```python
from build123d import *

# Parameters (mm, degrees)
F0_W     = 111
F0_H     = 68.5
F0_W_2   = 108
F0_H_2   = 65.5
F0_R     = 2.5
F0_R_2   = 1.25
F1_DEPTH = 1.5
F2_DEPTH = 13
F3_DEPTH = 8


with BuildPart() as f1:
    # F0 (on Top) → F1 (new body)
    with BuildSketch(Plane.XY):
        with Locations((-16, 1.25)):
            Rectangle(F0_W, F0_H)
        with Locations((-16, 1.25)):
            Rectangle(F0_W_2, F0_H_2, mode=Mode.SUBTRACT)
        with Locations((-16, 1.25)):
            Rectangle(F0_W_2, F0_H_2)
        with Locations((-34, -10.5)):
            Circle(F0_R, mode=Mode.SUBTRACT)
        with Locations((34, -10.5)):
            Circle(F0_R, mode=Mode.SUBTRACT)
        with Locations((-34, 27.1)):
            Circle(F0_R, mode=Mode.SUBTRACT)
        with Locations((34, 27.1)):
            Circle(F0_R, mode=Mode.SUBTRACT)
        with Locations((-34, -10.5)):
            Circle(F0_R)
        with Locations((-34, -10.5)):
            Circle(F0_R_2, mode=Mode.SUBTRACT)
        with Locations((-34, -10.5)):
            Circle(F0_R_2)
        with Locations((34, -10.5)):
            Circle(F0_R)
        with Locations((34, -10.5)):
            Circle(F0_R_2, mode=Mode.SUBTRACT)
        with Locations((34, -10.5)):
            Circle(F0_R_2)
        with Locations((34, 27.1)):
            Circle(F0_R)
        with Locations((34, 27.1)):
            Circle(F0_R_2, mode=Mode.SUBTRACT)
        with Locations((34, 27.1)):
            Circle(F0_R_2)
        with Locations((-34, 27.1)):
            Circle(F0_R)
        with Locations((-34, 27.1)):
            Circle(F0_R_2, mode=Mode.SUBTRACT)
        with Locations((-34, 27.1)):
            Circle(F0_R_2)
    extrude(amount=-F1_DEPTH)

    # F0 (on Top) → F2 (join)
    with BuildSketch(Plane.XY):
        with Locations((-16, 1.25)):
            Rectangle(F0_W, F0_H)
        with Locations((-16, 1.25)):
            Rectangle(F0_W_2, F0_H_2, mode=Mode.SUBTRACT)
        with Locations((-34, 27.1)):
            Circle(F0_R_2)
        with Locations((34, 27.1)):
            Circle(F0_R_2)
        with Locations((34, -10.5)):
            Circle(F0_R_2)
        with Locations((-34, -10.5)):
            Circle(F0_R_2)
    extrude(amount=F2_DEPTH)

    # F0 (on Top) → F3 (join)
    with BuildSketch(Plane.XY):
        with Locations((-34, 27.1)):
            Circle(F0_R)
        with Locations((-34, 27.1)):
            Circle(F0_R_2, mode=Mode.SUBTRACT)
        with Locations((-34, -10.5)):
            Circle(F0_R)
        with Locations((-34, -10.5)):
            Circle(F0_R_2, mode=Mode.SUBTRACT)
        with Locations((34, 27.1)):
            Circle(F0_R)
        with Locations((34, 27.1)):
            Circle(F0_R_2, mode=Mode.SUBTRACT)
        with Locations((34, -10.5)):
            Circle(F0_R)
        with Locations((34, -10.5)):
            Circle(F0_R_2, mode=Mode.SUBTRACT)
    extrude(amount=F3_DEPTH)


solid = f1.part
```
Geometry: final body of the model. Coordinates: model frame, mm. A direction names the side the tool comes from. Coordinates: 2 decimals unless noted, no trailing zeros. Order: outer loops, then holes, each group sorted by start corner. A loop starts at its lowest first (then second) coordinate and runs counter-clockwise, first axis right, second up. Notation, with made-up numbers: (-15.75, -2) - (18.25, -2) arc R8 cw to (18.25, 9) - close; hole circle Ø3 at (73, 61). An arc over 180 degrees is marked (long way). Write each question's results on one line, items separated by ' | '.
(1) Section query D-D, the plane y = -10.5. Return the cut outline in (x, z), plus the area to 4 significant figures.
Values found:
outline: (-71.5, -1.5) - (39.5, -1.5) - (39.5, 13) - (38, 13) - (38, 0) - (36.5, 0) - (36.5, 8) - (35.25, 8) - (35.25, 13) - (32.75, 13) - (32.75, 8) - (31.5, 8) - (31.5, 0) - (-31.5, 0) - (-31.5, 8) - (-32.75, 8) - (-32.75, 13) - (-35.25, 13) - (-35.25, 8) - (-36.5, 8) - (-36.5, 0) - (-70, 0) - (-70, 13) - (-71.5, 13) - close | area: 310.5 mm²
(2) Section query C-C, the plane x = -34. Return the cut outline in (y, z), plus the area to 3 significant figures.
Values found:
outline: (-33, -1.5) - (35.5, -1.5) - (35.5, 13) - (34, 13) - (34, 0) - (29.6, 0) - (29.6, 8) - (28.35, 8) - (28.35, 13) - (25.85, 13) - (25.85, 8) - (24.6, 8) - (24.6, 0) - (-8, 0) - (-8, 8) - (-9.25, 8) - (-9.25, 13) - (-11.75, 13) - (-11.75, 8) - (-13, 8) - (-13, 0) - (-31.5, 0) - (-31.5, 13) - (-33, 13) - close | area: 247 mm²
(3) First-contact query: pin 1 Ø1.5 at (x, y) = (16, 19.5) entering from +Z; pin 2 Ø1.5 at (x, y) = (-34.5, 28.5) entering from +Z. Flat tips, straight axial feed; report the tip coordinate or a pass-through.
Values found:
pin 1: stops at z = 0 | pin 2: stops at z = 13
(4) Set-up query: faces 1 (the face through (35, 26, 8)), 2 (the face through (-71.5, 1, 6)). Return all of +Z, -Z, +X, -X, +Y, -Y with unobstructed straight access to the full face (end or side cutting, diameter ignored); none if empty.
Values found:
face 1: +Z | face 2: +Z, -Z, -X, +Y, -Y
(5) Section query A-A, the plane z = 11. Return the cut outline in (x, y).
Values found:
outline: (-71.5, -33) - (39.5, -33) - (39.5, 35.5) - (-71.5, 35.5) - close; circle Ø2.5 at (-34, -10.5); circle Ø2.5 at (-34, 27.1); circle Ø2.5 at (34, -10.5); circle Ø2.5 at (34, 27.1); hole (-70, -31.5) - (38, -31.5) - (38, 34) - (-70, 34) - close
(6) Mould query, pull axis X, two halves, no side actions, for faces 3 (the face through (-17, -33, 6)), 4 (the face through (39.5, 1, 6)), 5 (the face through (-33, 26, 8)). Classes: +X half, -X half, draft (parallel to the pull), parting line (faces both ways), or undercut.
Values found:
face 3: draft | face 4: +X half | face 5: undercut
(7) Line query: line 1 (X direction, y = -17.5, z = 2); line 2 (Y direction, x = -13.5, z = 2.75); line 3 (Z direction, x = -14, y = 11.5). Output: solid intervals per line, ascending. Write a range as [from, to].
Values found:
line 1: x = [-71.5, -70], [38, 39.5] | line 2: y = [-33, -31.5], [34, 35.5] | line 3: z = [-1.5, 0]
(8) Section query B-B, the plane z = 4. Return the cut outline in (x, y), plus the area to 3 significant figures.
Values found:
outline: (-71.5, -33) - (39.5, -33) - (39.5, 35.5) - (-71.5, 35.5) - close; circle Ø5 at (-34, -10.5); circle Ø5 at (-34, 27.1); circle Ø5 at (34, -10.5); circle Ø5 at (34, 27.1); hole (-70, -31.5) - (38, -31.5) - (38, 34) - (-70, 34) - close | area: 608 mm²
